from build123d import *

# Parameters (mm, degrees)
SKETCH_1_W          = 300
SKETCH_1_H          = 145
EXTRUDE_1_DEPTH     = 81
SHELL_1_T           = -6
SKETCH_2_R          = 2.55
CUT_EXTRUDE_1_DEPTH = 183.705363906
SKETCH_3_R          = 4.25
CUT_EXTRUDE_2_DEPTH = 3


with BuildPart() as part:
    # ｽｹｯﾁ1 → ﾎﾞｽ - 押し出し1 (new body)
    with BuildSketch(Plane(origin=(0, 0, 0), x_dir=(1, 0, 0), z_dir=(0, 1, 0))):
        Rectangle(SKETCH_1_W, SKETCH_1_H)
    extrude(amount=EXTRUDE_1_DEPTH)

    # ｼｪﾙ1
    shell_1_openings = [part.faces().sort_by_distance(p)[0] for p in [
        (0, 81, 0),
    ]]
    offset(amount=SHELL_1_T, openings=shell_1_openings, kind=Kind.INTERSECTION)

    # ｽｹｯﾁ2 → ｶｯﾄ - 押し出し1 (cut, through all)
    with BuildSketch(Plane(origin=(0, 6, 0), x_dir=(1, 0, 0), z_dir=(0, 1, 0))):
        with Locations(Location((140, 60, 0), (0, 0, 270))):
            Circle(SKETCH_2_R)
        with Locations(Location((140, -60, 0), (0, 0, 90))):
            Circle(SKETCH_2_R)
        with Locations(Location((-22.5, -60, 0), (0, 0, 270))):
            Circle(SKETCH_2_R)
        with Locations(Location((-22.5, 60, 0), (0, 0, 90))):
            Circle(SKETCH_2_R)
    extrude(amount=-CUT_EXTRUDE_1_DEPTH, mode=Mode.SUBTRACT)

    # ｽｹｯﾁ3 → ｶｯﾄ - 押し出し2 (cut)
    with BuildSketch(Plane(origin=(0, 6, 0), x_dir=(1, 0, 0), z_dir=(0, 1, 0))):
        with Locations(Location((140, 60, 0), (0, 0, 270))):
            Circle(SKETCH_3_R)
        with Locations(Location((-22.5, 60, 0), (0, 0, 270))):
            Circle(SKETCH_3_R)
        with Locations(Location((-22.5, -60, 0), (0, 0, 270))):
            Circle(SKETCH_3_R)
        with Locations(Location((140, -60, 0), (0, 0, 270))):
            Circle(SKETCH_3_R)
    extrude(amount=-CUT_EXTRUDE_2_DEPTH, mode=Mode.SUBTRACT)


solid = part.part
Here's how the part is built. I have some questions about the finished solid (model axes, mm). A direction names the side the tool comes from. Coordinates: 2 decimals unless noted, no trailing zeros. Write each loop counter-clockwise with the first axis right and the second up, starting at its lowest first coordinate (ties: lowest second). Pieces come first, ordered by that corner, then holes. Notation, with made-up numbers: (-10.75, 53) - (-1.75, 53) arc R35 ccw to (-1.75, 92) - close; hole circle Ø2 at (78.25, 0). An arc over 180 degrees is marked (long way). Use one line per item in the form item = value.
1) Suppose I cut it at C-C, the plane z = -30. Write out the boundary of the cut face in (x, y), plus the area to 3 significant figures.
Solved:
outline = (-150, 0) - (150, 0) - (150, 81) - (144, 81) - (144, 6) - (-144, 6) - (-144, 81) - (-150, 81) - close
area = 2,700 mm2
2) On a 3-axis mill with a long thin cutter (end or side, diameter ignored), from which of +Z, -Z, +X, -X, +Y, -Y can I reach the whole of each face in a straight line? I mean faces 1 (the flat face through (-2, 6, -1)), 2 (the flat face through (-2, 0, -1)). Say none if no direction works.
Solved:
face_1 = +Y
face_2 = +Z, -Z, +X, -X, -Y
3) Suppose I cut it at A-A, the plane y = 38. Write out the boundary of the cut face in (x, z), plus the area to 3 significant figures.
Solved:
outline = (-150, -72.5) - (150, -72.5) - (150, 72.5) - (-150, 72.5) - close; hole (-144, -66.5) - (144, -66.5) - (144, 66.5) - (-144, 66.5) - close
area = 5,200 mm2
4) I need wall thicknesses on line 1 (X direction, y = 1, z = 60); line 2 (X direction, y = 4.1, z = -60); line 3 (Z direction, x = 140, y = 1.25). Which ranges of each line are inside material? Lowest first, please.
Solved:
line_1 = -150 to -25.05, -19.95 to 137.45, 142.55 to 150
line_2 = -150 to -26.75, -18.25 to 135.75, 144.25 to 150
line_3 = -72.5 to -62.55, -57.45 to 57.45, 62.55 to 72.5
5) I'm going to push a flat-ended pin straight in: P1, Ø5, axis at x = -82, z = 3, coming from the +Y side. Where does the tip first touch, or does it pass through?
Solved:
P1 = 6
6) Suppose I cut it at B-B, the plane x = 74. Write out the boundary of the cut face in (y, z), plus the area to 3 significant figures.
Solved:
outline = (0, -72.5) - (81, -72.5) - (81, -66.5) - (6, -66.5) - (6, 66.5) - (81, 66.5) - (81, 72.5) - (0, 72.5) - close
area = 1,770 mm2
7) Thinking about a two-plate mould opening in Z: for faces 3 (the cylindrical face through (-24.128, 4.521, 63.926)), 4 (the flat face through (-150, 40, 1)), 5 (the flat face through (-2, 40, 72.5)), which applies, released by +Z, released by -Z, zero draft, split by the parting line, or undercut?
Solved:
face_3 = undercut
face_4 = zero draft
face_5 = released by +Z
